```python
from build123d import *

# Parameters (mm, degrees)
SKETCH1_R           = 10
BOSS_EXTRUDE1_DEPTH = 20


with BuildPart() as part:
    # Sketch1 → Boss-Extrude1 (new body)
    with BuildSketch(Plane(origin=(0, 0, 0), x_dir=(1, 0, 0), z_dir=(0, 1, 0))):
        with BuildLine():
            Line((5.103736684, -12.52406407), (20, -12.52406407))
            Line((20, -12.52406407), (20, -14.52406407))
            Line((20, -14.52406407), (-20, -14.52406407))
            Line((-20, -14.52406407), (-20, -12.52406407))
            Line((-20, -12.52406407), (-5.103736684, -12.52406407))
            ThreePointArc((-5.103736684, -12.52406407), (0, 13.52406407), (5.103736684, -12.52406407))
        make_face()
        with Locations(Location((0, 0, 0), (0, 0, 270))):
            Circle(SKETCH1_R, mode=Mode.SUBTRACT)
    extrude(amount=BOSS_EXTRUDE1_DEPTH)


solid = part.part
```
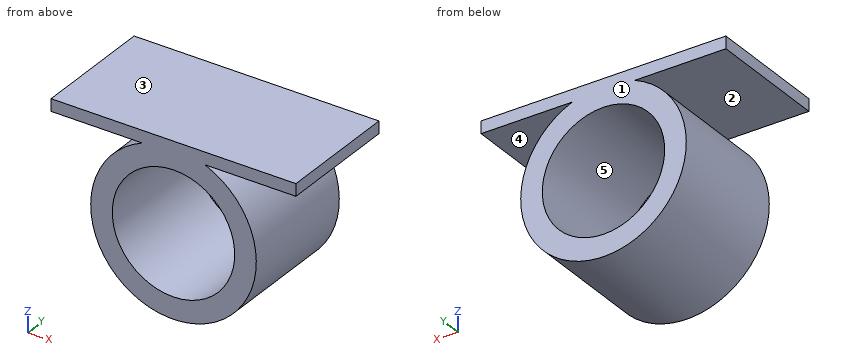
For this review, take the finished solid that the model builds, in its own axes (mm). Face numbers are marked on the shaded views. A direction names the side the tool comes from. Coordinates: 2 decimals unless noted, no trailing zeros. Write each loop counter-clockwise with the first axis right and the second up, starting at its lowest first coordinate (ties: lowest second). Pieces come first, ordered by that corner, then holes.
(1) The part is to be moulded in two halves that separate along Z. For the marked faces 1, 2 and 3, say which applies: +Z half, -Z half, draft (parallel to the pull), parting line (faces both ways), or undercut.
(2) Add section B-B on z = 0. Give the boundary of the cut face in (x, y), then the cut area to 3 significant figures.
(3) Tool access review of the marked faces 4 and 5: name each direction out of +Z, -Z, +X, -X, +Y, -Y from which nothing blocks a thin tool from reaching the whole face with its end or side.
(4) Wall thickness on probe 1 along X at (y, z) = (6.75, 0); probe 2 along Z at (x, y) = (-15.5, 17.5); probe 3 along X at (y, z) = (7, -7): over which ranges is each line inside the solid? List them lowest first.
(5) For pin 1 Ø2 at (y, z) = (11.5, 0) entering from -X; pin 2 Ø2 at (y, z) = (13, 11) entering from +X; pin 3 Ø7.5 at (x, y) = (9.5, 6.5) entering from -Z, all flat-tipped, find the tip position at first contact; note any pin that passes through.
(6) Add section A-A on x = 0. Give the boundary of the cut face in (y, z), then the cut area to 3 significant figures.
(7) Add section C-C on y = 7.75. Give the boundary of the cut face in (x, z), then the cut area to 3 significant figures.
(8) Add section D-D on x = 7. Give the boundary of the cut face in (y, z).
Answer sheet:
1. face 1: draft
1. face 2: undercut
1. face 3: +Z half
2. outline: (-13.52, 0) - (-10, 0) - (-10, 20) - (-13.52, 20) - close; (10, 0) - (13.52, 0) - (13.52, 20) - (10, 20) - close
2. area: 141 mm2
3. face 4: +X, +Y, -Y
3. face 5: +Y, -Y
4. probe 1: x = -13.52 to -10, 10 to 13.52
4. probe 2: z = 12.52 to 14.52
4. probe 3: x = -11.57 to -7.14, 7.14 to 11.57
5. pin 1: stops at x = -13.52
5. pin 2: stops at x = 9.1
5. pin 3: stops at z = -12.24
6. outline: (0, -13.52) - (20, -13.52) - (20, -10) - (0, -10) - close; (0, 10) - (20, 10) - (20, 14.52) - (0, 14.52) - close
6. area: 161 mm2
7. outline: (-20, 12.52) - (-5.1, 12.52) arc R13.52 ccw (long way) to (5.1, 12.52) - (20, 12.52) - (20, 14.52) - (-20, 14.52) - close; hole circle Ø20 at (0, 0)
7. area: 334 mm2
8. outline: (0, -11.57) - (20, -11.57) - (20, -7.14) - (0, -7.14) - close; (0, 7.14) - (20, 7.14) - (20, 11.57) - (0, 11.57) - close; (0, 12.52) - (20, 12.52) - (20, 14.52) - (0, 14.52) - close
